from build123d import *

# Parameters (mm, degrees)
EXTRUDE_1_DEPTH     = 2
EXTRUDE_1_2_DEPTH   = 15
SKETCH_4_R          = 2
CUT_EXTRUDE_1_DEPTH = 15
SKETCH_5_R          = 2
CUT_EXTRUDE_2_DEPTH = 283


with BuildPart() as part:
    # 草图1 → Extrude 1 (new body)
    with BuildSketch(Plane.XY):
        with BuildLine():
            Line((0, 53.35), (-208, 53.35))
            ThreePointArc((-208, 53.35), (-209.414213562, 52.764213562), (-210, 51.35))
            Line((-210, 51.35), (-210, -241.65))
            ThreePointArc((-210, -241.65), (-209.414213562, -243.064213562), (-208, -243.65))
            Line((-208, -243.65), (-2, -243.65))
            ThreePointArc((-2, -243.65), (-0.585786438, -243.064213562), (0, -241.65))
            Line((0, -241.65), (0, -32.65))
            ThreePointArc((0, -32.65), (43, 10.35), (0, 53.35))
        make_face()
    extrude(amount=EXTRUDE_1_DEPTH)

    # 草图3 → Extrude 1 2 (add)
    with BuildSketch(Plane(origin=(0, 0, 0), x_dir=(-1, 0, 0), z_dir=(0, 0, -1))):
        Polygon((207.2, 48.687657947), (207.2, -238.454577256), (205.130446753, -240.85), (5.682615129, -240.85), (2.8, -238.359531245), (2.8, -37.127932812), (5.8, -37.127932812), (5.8, -236.986839537), (6.799072726, -237.85), (203.757755045, -237.85), (204.2, -237.338119658), (204.2, 48.687657947), align=None)
    extrude(amount=EXTRUDE_1_2_DEPTH)

    # 草图4 → 切除-拉伸1 (cut)
    with BuildSketch(Plane.XZ.offset(240.85)):
        with Locations((-167.807888651, -7.5)):
            Circle(SKETCH_4_R)
        with Locations((-42.192111349, -7.5)):
            Circle(SKETCH_4_R)
    extrude(amount=-CUT_EXTRUDE_1_DEPTH, mode=Mode.SUBTRACT)

    # 草图5 → 切除-拉伸2 (cut)
    with BuildSketch(Plane.ZY.offset(207.2)):
        with Locations((-7.5, -190.350496004)):
            Circle(SKETCH_5_R)
        with Locations((-7.5, -84.801056957)):
            Circle(SKETCH_5_R)
    extrude(amount=-CUT_EXTRUDE_2_DEPTH, mode=Mode.SUBTRACT)


solid = part.part
Here's how the part is built. I have some questions about the finished solid (model axes, mm). A direction names the side the tool comes from. Round coordinates to 2 decimals unless told otherwise and drop trailing zeros. Write each loop counter-clockwise with the first axis right and the second up, starting at its lowest first coordinate (ties: lowest second). Pieces come first, ordered by that corner, then holes. Notation, with made-up numbers: (-5, -13.75) -> (6, -13.75) arc R13 cw to (6, -9.75) -> close; hole circle Ø2 at (40.5, 85.5). An arc over 180 degrees is marked (long way). One line per item, written item: value.
1) Suppose I cut it at B-B on z = -12.25. List the corners of the cut face in (x, y) for me, plus the area to 3 significant figures.
Filled sheet:
outline: (-207.2, -238.45) -> (-205.13, -240.85) -> (-5.68, -240.85) -> (-2.8, -238.36) -> (-2.8, -37.13) -> (-5.8, -37.13) -> (-5.8, -236.99) -> (-6.8, -237.85) -> (-203.76, -237.85) -> (-204.2, -237.34) -> (-204.2, 48.69) -> (-207.2, 48.69) -> close
area: 2,070 mm2
2) Suppose I cut it at A-A on x = -155.5. List the corners of the cut face in (y, z) for me, plus the area to 3 significant figures.
Filled sheet:
outline: (-243.65, 0) -> (-240.85, 0) -> (-240.85, -15) -> (-237.85, -15) -> (-237.85, 0) -> (53.35, 0) -> (53.35, 2) -> (-243.65, 2) -> close
area: 639 mm2
3) Suppose I cut it at D-D on y = -53.5. List the corners of the cut face in (x, z) for me.
Filled sheet:
outline: (-210, 0) -> (-207.2, 0) -> (-207.2, -15) -> (-204.2, -15) -> (-204.2, 0) -> (-5.8, 0) -> (-5.8, -15) -> (-2.8, -15) -> (-2.8, 0) -> (0, 0) -> (0, 2) -> (-210, 2) -> close
4) If I drill on line 1 (Y direction, x = -3.8, z = -7.5); line 2 (X direction, y = -53.5, z = -11.75); line 3 (Y direction, x = -206, z = -7.5), over which ranges is the centre line in solid material (lowest first)? Write a range as [from, to].
Filled sheet:
line 1: y = [-239.22, -192.35], [-188.35, -86.8], [-82.8, -37.13]
line 2: x = [-207.2, -204.2], [-5.8, -2.8]
line 3: y = [-239.84, -192.35], [-188.35, -86.8], [-82.8, 48.69]
5) For faces 5 (the face through (-2.8, -139, -7)), 6 (the face through (-5.8, -136, -7)), 7 (the face through (-107, -240.85, -7)), 8 (the face through (-85, -93, 2)), which set-ups out of +Z, -Z, +X, -X, +Y, -Y let a thin tool reach every point of the face, with its end or its side?
Filled sheet:
face 5: -Z, +X, +Y, -Y
face 6: -Z, +Y
face 7: -Z, +X, -X, -Y
face 8: +Z, +X, -X, +Y, -Y
6) Suppose I cut it at C-C on y = 10.35. List the corners of the cut face in (x, z) for me, plus the area to 3 significant figures.
Filled sheet:
outline: (-210, 0) -> (-207.2, 0) -> (-207.2, -15) -> (-204.2, -15) -> (-204.2, 0) -> (43, 0) -> (43, 2) -> (-210, 2) -> close
area: 551 mm2
7) We'd pull the mould along X, two halves only. Please class faces 1 (the face through (-207.2, -93, -7)), 2 (the face through (-104, -237.85, -7)), 3 (the face through (-204.2, -96, -7)), 4 (the face through (42.99, 9.4, 0.99)): released by +X, released by -X, zero draft, split by the parting line, or undercut.
Filled sheet:
face 1: released by -X
face 2: undercut
face 3: undercut
face 4: released by +X
8) I'm going to push flat-ended pins straight in: pin 1 Ø4.5 at (y, z) = (-109, -10.5) entering from -X; pin 2 Ø6.5 at (x, z) = (-167.81, -7.5) entering from +Y; pin 3 Ø5 at (y, z) = (-123, -6) entering from +X. Where does each tip first touch, or does it pass through?
Filled sheet:
pin 1: stops at x = -207.2
pin 2: stops at y = -237.85
pin 3: stops at x = -2.8
